Geometry check sheet. Reference: the model listing, model coordinates, mm. A direction names the side the tool comes from. Give positions to 0.01 mm unless a question says otherwise; leave off trailing zeros. Order: outer loops, then holes, each group sorted by start corner. A loop starts at its lowest first (then second) coordinate and runs counter-clockwise, first axis right, second up. Notation, with made-up numbers: M 2,11 L 42,11 A21 cw 42,34 Z; hole C 43,-31 d9. An arc over 180 degrees is marked long. Put each result on its own line as item: value. Start each with the question number.
Q1. Section check A-A on z = -3.75. Record the cut outline in (x, y), then the cut area to 3 significant figures.
Q2. Section check C-C on y = 27.75. Record the cut outline in (x, z).
Q3. Section check B-B on x = -10. Record the cut outline in (y, z).
Q4. Mould release check, pull along Y, two halves, no side actions. Record for faces 1 (the flat face through (14, 6, 0)), 2 (the flat face through (10, 22.8, 5)), 3 (the flat face through (13.9, 16, 1.5)), 4 (the flat face through (16.25, 17, 3)): +Y half, -Y half, draft (parallel to the pull), parting line (faces both ways), or undercut.
Q5. Go/stop test with flat-tipped pins: pin 1 (3.5 mm diameter, centred on x = 14.025, z = 0, fed in from -Y); pin 2 (4.5 mm diameter, centred on y = 20, z = 2.5, fed in from +X); pin 3 (6.5 mm diameter, centred on y = 10.5, z = 0.5, fed in from +X). Record where each tip stops, or that it passes through.
Q6. Section check D-D on x = -1. Record the cut outline in (y, z).
Q7. Material ranges on L1, parallel to X at y = 18.15, z = 0; L2, parallel to Y at x = -1, z = 3.5; L3, parallel to X at y = 15, z = 2.5, recorded low to high.
Q8. Access from +Z, -Z, +X, -X, +Y, -Y to the whole of each face (thin tool, end or side, straight path). Record for faces 5 (the flat face through (-16, 17, 0.6)), 6 (the cylindrical face through (11.396, 24.723, 0.233)), 7 (the flat face through (11.4, 21, 0)).
```python
from build123d import *

# Parameters (mm, degrees)
BODY_DEPTH     = 6.3
HUB_BODY_DEPTH = 3.9
HUB_START      = -26.7
SKETCH3_R      = 2.56
HUB_DEPTH      = 30
HOLES_REACH    = 27.526
SKETCH5_W      = 4
SKETCH5_H      = 2
WIRES_2_DEPTH  = 6


with BuildPart() as part:
    # front body → body (new, symmetric)
    with BuildSketch(Plane.XY):
        Polygon((-11.4, 22.8), (11.4, 22.8), (11.4, 18.65), (16.25, 18.65), (16.25, 16), (11.4, 16), (11.4, 0), (-11.4, 0), (-11.4, 16), (-16.25, 16), (-16.25, 18.65), (-11.4, 18.65), align=None)
    extrude(amount=BODY_DEPTH, both=True)

    # Sketch2 → hub body (add)
    with BuildSketch(Plane(origin=(0, 22.8, 0), x_dir=(1, 0, 0), z_dir=(0, 1, 0))):
        with BuildLine():
            ThreePointArc((-0.442105263, -2.995841994), (11.4, 0), (-0.442105263, 2.995841994))
            ThreePointArc((-0.442105263, 2.995841994), (-3.6, 0), (-0.442105263, -2.995841994))
        make_face()
    extrude(amount=HUB_BODY_DEPTH)

    # Sketch3 → hub (add)
    with BuildSketch(Plane(origin=(0, 26.7, 0), x_dir=(1, 0, 0), z_dir=(0, 1, 0)).offset(HUB_START)):
        with Locations(Location((5.1, 0, 0), (0, 0, 270))):
            Circle(SKETCH3_R)
    extrude(amount=HUB_DEPTH)

    # mounting holes → holes (cut, up to next)
    with BuildSketch(Plane(origin=(0, 18.65, 0), x_dir=(1, 0, 0), z_dir=(0, 1, 0)), mode=Mode.PRIVATE) as holes_sk1:
        with BuildLine():
            Line((-14.976643316, 0.6), (-16.25, 0.6))
            Line((-16.25, 0.6), (-16.25, -0.6))
            Line((-16.25, -0.6), (-14.976643316, -0.6))
            ThreePointArc((-14.976643316, -0.6), (-12.9, 0), (-14.976643316, 0.6))
        make_face()
    holes_tool1 = extrude(holes_sk1.sketch, amount=-HOLES_REACH, mode=Mode.PRIVATE) & part.part
    # mounting holes → holes (cut, up to next)
    with BuildSketch(Plane(origin=(0, 18.65, 0), x_dir=(1, 0, 0), z_dir=(0, 1, 0)), mode=Mode.PRIVATE) as holes_sk2:
        with BuildLine():
            Line((16.25, 0.6), (16.25, -0.6))
            Line((16.25, -0.6), (14.976643316, -0.6))
            ThreePointArc((14.976643316, -0.6), (12.9, 0), (14.976643316, 0.6))
            Line((14.976643316, 0.6), (16.25, 0.6))
        make_face()
    holes_tool2 = extrude(holes_sk2.sketch, amount=-HOLES_REACH, mode=Mode.PRIVATE) & part.part
    add(holes_tool1.solids().sort_by_distance((-14.450684, 18.65, 0))[0], mode=Mode.SUBTRACT)
    add(holes_tool2.solids().sort_by_distance((14.450684, 18.65, 0))[0], mode=Mode.SUBTRACT)

    # Sketch5 → Wires 2 (add)
    with BuildSketch(Plane(origin=(11.4, 0, 0), x_dir=(0, 0, -1), z_dir=(1, 0, 0))):
        with Locations((0, 5)):
            Rectangle(SKETCH5_W, SKETCH5_H)
    extrude(amount=WIRES_2_DEPTH)


solid = part.part
```
Results found:
1. outline: M -16.25,16 L -11.4,16 L -11.4,0 L 11.4,0 L 11.4,16 L 16.25,16 L 16.25,18.65 L 11.4,18.65 L 11.4,22.8 L 10.16,22.8 L 10.16,26.7 L 0.04,26.7 L 0.04,22.8 L -11.4,22.8 L -11.4,18.65 L -16.25,18.65 Z
1. area: 585 mm^2
2. outline: C 5.1,0 d5.12
3. outline: M 0,-6.3 L 22.8,-6.3 L 22.8,6.3 L 0,6.3 Z
4. face 1: undercut
4. face 2: +Y half
4. face 3: undercut
4. face 4: draft
5. pin 1: stops at y = 4
5. pin 2: stops at x = 16.25
5. pin 3: stops at x = 11.4
6. outline: M 0,-6.3 L 22.8,-6.3 L 22.8,-2.97 L 26.7,-2.97 L 26.7,2.97 L 22.8,2.97 L 22.8,6.3 L 0,6.3 Z
7. L1: x = -12.9 to 12.9
7. L2: y = 0 to 22.8
7. L3: x = -11.4 to 11.4
8. face 5: -X, +Y, -Y
8. face 6: +Y
8. face 7: +Z, -Z, +X, +Y
